Design review of the part shown in the three views and the two pictorial views. Dimensions are in mm from the part's minimum x, y and z. A direction names the side the tool comes from. Round coordinates to 2 decimals unless told otherwise and drop trailing zeros. Order: outer loops, then holes, each group sorted by start corner. A loop starts at its lowest first (then second) coordinate and runs counter-clockwise, first axis right, second up. Notation, with made-up numbers: M 80.25,-28.75 L 98.25,-28.75 A13 cw 98.25,-10.75 Z; hole C -7,-1.75 d2. An arc over 180 degrees is marked long. Write each question's results on one line, items separated by ' | '. Start each with the question number.
Item 1: Clearance check with flat-ended pins moving along their axes: pin 1 (10 mm diameter, centred on x = 17, y = 12, fed in from +Z); pin 2 (3 mm diameter, centred on x = 13.5, y = 4.5, fed in from -Z); pin 3 (1 mm diameter, centred on x = 25.5, y = 12, fed in from -Z). State where each tip first meets the part, or that it passes through.
Item 2: Take a section at A-A, the plane z = 23. Write out the cut boundary in (x, y).
Item 3: Machinability: for the marked faces 1, 2, 3, 4 and 5, which of the approach directions +Z, -Z, +X, -X, +Y, -Y give a long, thin tool a straight path to every point of the face, cutting with its end or side? Answer none if there is none.
Item 4: The part is to be moulded in two halves that separate along X. For the marked faces 6, 7, 8 and 9, say which applies: +X half, -X half, draft (parallel to the pull), parting line (faces both ways), or undercut.
Item 5: Take a section at B-B, the plane y = 2. Write out the cut boundary in (x, z).
Item 6: Wall thickness on line 1 (X direction, y = 19.5, z = 18); line 2 (X direction, y = 12.5, z = 21.75); line 3 (Z direction, x = 25.25, y = 12.25) (3 decimals): over which ranges is each line inside the solid? List them lowest first. Write a range as [from, to].
Item 7: Take a section at D-D, the plane z = 10. Write out the cut boundary in (x, y).
Item 8: Take a section at C-C, the plane y = 14.5. Write out the cut boundary in (x, z) (3 decimals).
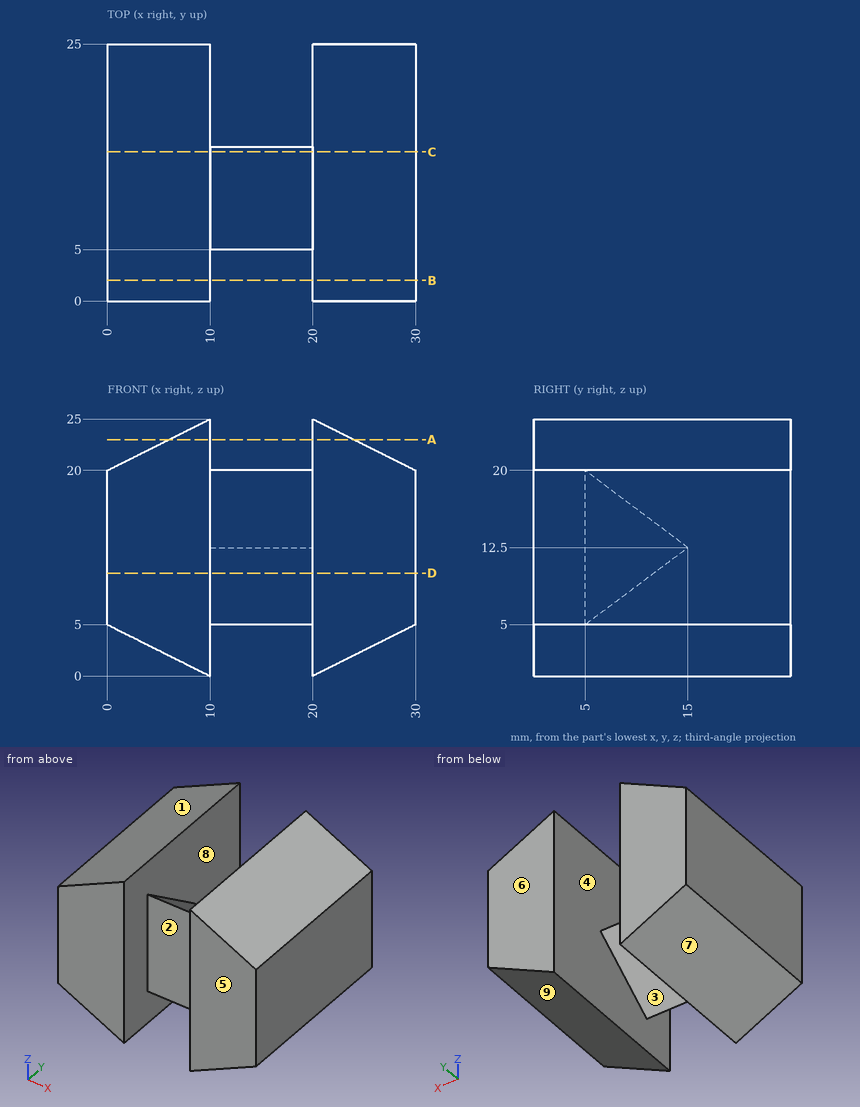
Results list:
1) pin 1: z = 25 | pin 2: z = 5 | pin 3: z = 2.5
2) outline: M 6,0 L 10,0 L 10,25 L 6,25 Z; M 20,0 L 24,0 L 24,25 L 20,25 Z
3) face 1: +Z, -X, +Y, -Y | face 2: +Z, -Z, -Y | face 3: -Z, +Y | face 4: none | face 5: +Z, -Z, +X, -X, -Y
4) face 6: draft | face 7: -X half | face 8: undercut | face 9: +X half
5) outline: M 0,5 L 10,0 L 10,25 L 0,20 Z; M 20,0 L 30,5 L 30,20 L 20,25 Z
6) line 1: [0, 10], [20, 30] | line 2: [3.5, 10], [20, 26.5] | line 3: [2.625, 22.375]
7) outline: M 0,0 L 10,0 L 10,5 L 20,5 L 20,0 L 30,0 L 30,25 L 20,25 L 20,11.67 L 10,11.67 L 10,25 L 0,25 Z
8) outline: M 0,5 L 10,0 L 10,12.125 L 20,12.125 L 20,0 L 30,5 L 30,20 L 20,25 L 20,12.875 L 10,12.875 L 10,25 L 0,20 Z
